Autodesk Inventor part; units mm, degrees
ref_plane "YZ Plane" through (0, 0, 0) normal (1, 0, 0) x (0, 1, 0)
ref_plane "XZ Plane" through (0, 0, 0) normal (0, 1, 0) x (-1, 0, 0)
ref_plane "XY Plane" through (0, 0, 0) normal (0, 0, 1) x (1, 0, 0)
sketch "Sketch1" plane through (0, 0, 0) normal (1, 0, 0) x (0, 1, 0)
  line L0 (0, 95) -> (8.4, 95)
  line L1 (8.4, 95) -> (12, 81.5646)
  line L2 (12, 81.5646) -> (12, 0)
  line L3 (12, 0) -> (0, 0)
  line L4 (0, 0) -> (0, 73.5)
  line L5 (0, 73.5) -> (3.5, 73.5)
  line L6 (3.5, 73.5) -> (3.5, 76.5)
  line L7 (3.5, 76.5) -> (0, 76.5)
  line L8 (0, 76.5) -> (0, 95)
  line L9 (0, 114) -> (0, -19) construction
  line L10 (-2.4, 0) -> (14.4, 0)
  dimension "d0" = 95
  dimension "d1" = 12
  dimension "d2" = 8.4
  dimension "d3" = 3.5
  dimension "d4" = 3
  dimension "d5" = 73.5
  dimension "d6" = 165
revolve "Revolution1" add sketch "Sketch1" angle 360 about axis through (0, -10, 0) along (0, 1, 0)
sketch "Sketch2" plane through (0, 0, 0) normal (0, -1, 0) x (1, 0, 0)
  circle A0 centre (0, 0) radius 81.5646
  circle A1 centre (0, 0) radius 22
  circle A2 centre (0, 60) radius 10
  dimension "d8" = 44
  dimension "d9" = 20
  dimension "d10" = 60
extrude "Extrusion1" cut sketch "Sketch2" against normal through all contours A1 | A2
properties part number "top_flange"
Part model, mm, in its own coordinate system. A direction names the side the tool comes from. Round coordinates to 2 decimals unless told otherwise and drop trailing zeros. Order: outer loops, then holes, each group sorted by start corner. A loop starts at its lowest first (then second) coordinate and runs counter-clockwise, first axis right, second up. Notation, with made-up numbers: M -39.5,41.5 L 18.5,41.5 A26 ccw 18.5,67.5 Z; hole C -23.75,9 d10. An arc over 180 degrees is marked long. Put each result on its own line as item: value. Start each with the question number.
1. Drop flat-ended pins along their axis: pin 1 (1.5 mm diameter, centred on y = 2.5, z = -44.5, fed in from -X); pin 2 (1.5 mm diameter, centred on x = -31, y = 2.5, fed in from -Z). Give the stop position or say it passes through.
2. Slice it at A-A on z = 0. List the corners of the cut face in (x, y), then the cut area to 3 significant figures.
3. Drill centre lines: probe 1 along Z at (x, y) = (-8, 8.25); probe 2 along Z at (x, y) = (55.5, 3.25); probe 3 along Z at (x, y) = (-14, 3.75). Where is each one in solid material? Low to high. Write a range as [from, to].
4. Slice it at B-B on x = 0. List the corners of the cut face in (y, z), then the cut area to 3 significant figures.
5. Tool access for faces 1 (the face through (-24.752, 11.775, 78.6)), 2 (the face through (-71.752, 1.774, -15.933)): list every direction of +Z, -Z, +X, -X, +Y, -Y with a clear straight run to the whole face (end or side of a thin tool).
Findings:
1. pin 1: x = -84.33
1. pin 2: z = -90.06
2. outline: M -95,0 L -76.5,0 L -76.5,3.5 L -73.5,3.5 L -73.5,0 L -22,0 L -22,12 L -81.56,12 L -95,8.4 Z; M 22,0 L 73.5,0 L 73.5,3.5 L 76.5,3.5 L 76.5,0 L 95,0 L 95,8.4 L 81.56,12 L 22,12 Z
2. area: 1,680 mm2
3. probe 1: [-94.66, -20.49], [20.49, 54], [66, 94.66]
3. probe 2: [-77.1, -52.65], [-48.19, 48.19], [52.65, 77.1]
3. probe 3: [-93.96, -16.97], [16.97, 93.96]
4. outline: M 0,-95 L 8.4,-95 L 12,-81.56 L 12,-22 L 0,-22 L 0,-73.5 L 3.5,-73.5 L 3.5,-76.5 L 0,-76.5 Z; M 0,22 L 12,22 L 12,50 L 0,50 Z; M 0,70 L 12,70 L 12,81.56 L 8.4,95 L 0,95 L 0,76.5 L 3.5,76.5 L 3.5,73.5 L 0,73.5 Z
4. area: 1,440 mm2
5. face 1: +Y
5. face 2: -Y
